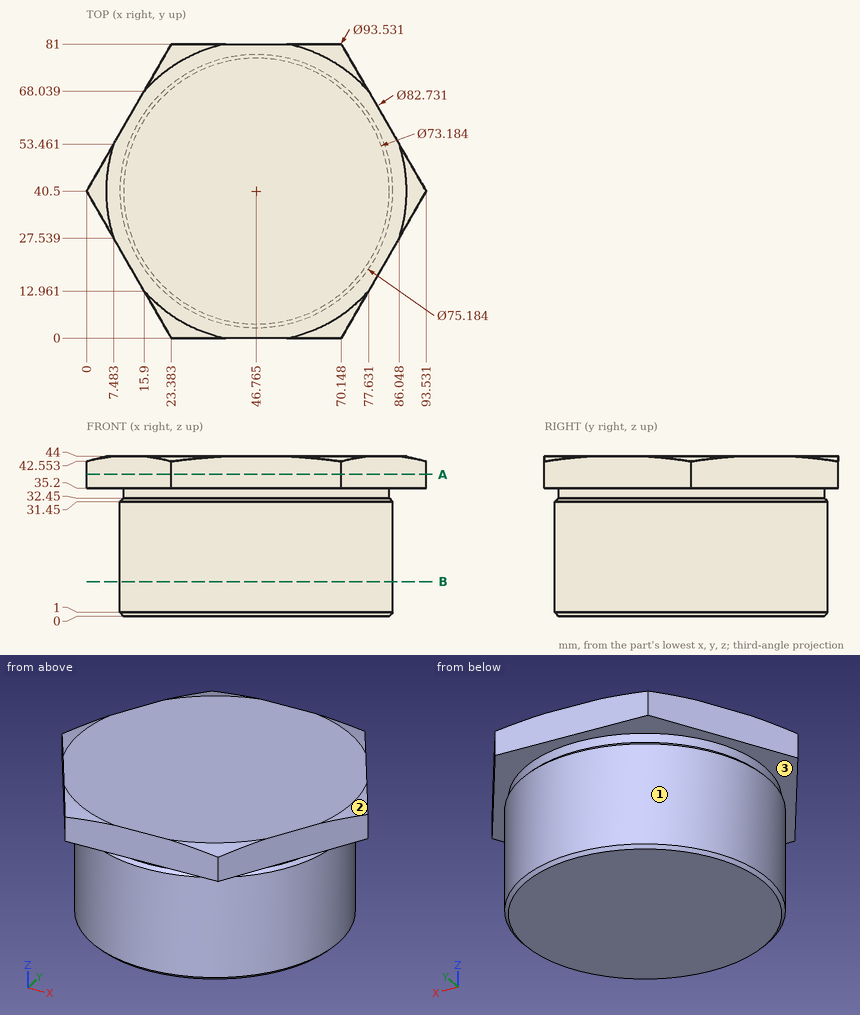
The drawing under review shows one solid part. Ordinate dimensions are in mm from its lowest x, y, z. A direction names the side the tool comes from. Give positions to 0.01 mm unless a question says otherwise; leave off trailing zeros. Write each loop counter-clockwise with the first axis right and the second up, starting at its lowest first coordinate (ties: lowest second). Pieces come first, ordered by that corner, then holes. Notation, with made-up numbers: (43, 70.25) -> (94, 70.25) arc R21 ccw to (94, 74.25) -> close; hole circle Ø2 at (-19.5, 60.25). An arc over 180 degrees is marked (long way). Use CSV: the item, a comma, the result in double quotes.
Q1. Take a section at B-B, the plane z = 9.5. Write out the cut boundary in (x, y) (1 decimal).
Conclusion:
outline,"circle Ø75.2 at (46.8, 40.5)"
Q2. Tool access review of the marked faces 1, 2 and 3: name each direction out of +Z, -Z, +X, -X, +Y, -Y from which nothing blocks a thin tool from reaching the whole face with its end or side.
Conclusion:
face 1,"-Z"
face 2,"+Z, +X"
face 3,"none"
Q3. To check wall thickness, follow probe 1 along Z at (x, y) = (85, 38); probe 2 along X at (y, z) = (39.5, 21.5); probe 3 along Z at (x, y) = (67, 71.5). State the ranges of each line that lie inside material, in increasing order. Write a range as [from, to].
Conclusion:
probe 1,"[35.2, 44]"
probe 2,"[9.19, 84.34]"
probe 3,"[0.43, 32.02], [35.2, 44]"
Q4. For P1, Ø6, axis at x = 33.5, z = 11.5, coming from the +Y side; P2, Ø3, axis at y = 67, z = 13.5, coming from the +X side; P3, Ø5, axis at x = 31.5, z = 32, coming from the -Y side, all flat-tipped, find the tip position at first contact; note any pin that passes through.
Conclusion:
P1,"y = 76.66"
P2,"x = 74.84"
P3,"y = 5.16"
Q5. Take a section at A-A, the plane z = 39. Write out the cut boundary in (x, y), then the cut area to 3 significant figures.
Conclusion:
outline,"(0, 40.5) -> (23.38, 0) -> (70.15, 0) -> (93.53, 40.5) -> (70.15, 81) -> (23.38, 81) -> close"
area,"5,680 mm2"
